Source: CAD feature listing. Evaluate the final solid. Frame: model axes, mm. A direction names the side the tool comes from. Round coordinates to 2 decimals unless told otherwise and drop trailing zeros. Order: outer loops, then holes, each group sorted by start corner. A loop starts at its lowest first (then second) coordinate and runs counter-clockwise, first axis right, second up. Notation, with made-up numbers: (52, -7) -> (108, -7) arc R19 cw to (108, 24) -> close; hole circle Ø8 at (-30, 86.5). An arc over 180 degrees is marked (long way). Write item = value, one per line. Start each with the question number.
(1) Cut plane B-B on x = 40. Return the cut outline in (y, z), then the cut area to 3 significant figures.
(2) Cut plane D-D on x = 12.5. Return the cut outline in (y, z).
(3) Cut plane C-C on z = -70. Return the cut outline in (x, y), then the cut area to 3 significant figures.
(4) Ray query, line 1 (Z direction, x = 40, y = 3); line 2 (Y direction, x = 5, z = -85); line 3 (Z direction, x = 17, y = 24). Return the intervals inside material, ascending.
(5) Contact query for flat-ended pins moving along their axis: pin 1 Ø6 at (x, z) = (40, -70) entering from +Y; pin 2 Ø8 at (x, z) = (24.5, -25.5) entering from -Y; pin 3 Ø1.5 at (x, z) = (39.5, -70) entering from -Y; pin 4 Ø10 at (y, z) = (35.5, -85.5) entering from +X. Output: stop coordinate, or through.
(6) Reachability of faces 1 (the face through (20, 5, -90)), 2 (the face through (25, 0, -49)) from +Z, -Z, +X, -X, +Y, -Y: full face, straight path, thin tool, end or side. Return the list, or none.
(7) Cut plane A-A on y = 4. Return the cut outline in (x, z).
(8) Draft query along X for faces 3 (the face through (42.31, 2.46, -70.96)), 4 (the face through (17.5, 2.5, -49.9)), 5 (the face through (50, 12, -49)), 6 (the face through (25, 12, -100)). Return one class per face: released by +X, released by -X, zero draft, split by the parting line, or undercut.
Autodesk Inventor part; units mm, degrees
ref_plane "Work Plane1" through (0, 55, 0) normal (0, 1, 0) x (1, 0, 0)
ref_plane "YZ Plane" through (0, 0, 0) normal (1, 0, 0) x (0, 1, 0)
ref_plane "XZ Plane" through (0, 0, 0) normal (0, 1, 0) x (-1, 0, 0)
sketch "Sketch1" plane through (0, 0, 0) normal (0, 1, 0) x (-1, 0, 0)
  line L0 (0, 0) -> (-50, 0)
  line L1 (-50, 0) -> (-50, -100)
  line L2 (-50, -100) -> (0, -100)
  line L3 (0, -100) -> (0, 0)
  dimension "d3" = 100
  dimension "d4" = 50
extrude "Extrusion1" add sketch "Sketch1" along normal blind 25
fillet "Fillet1" radius 2 1 edges at (25, 25, 0)
ref_plane "Work Plane1" through (0, 55, 0) normal (0, 1, 0) x (1, 0, 0)
sketch "Sketch2" plane through (0, 55, 0) normal (0, 1, 0) x (1, 0, 0)
  point P0 (0, 0)
sketch "Sketch3" plane through (0, 25, 0) normal (0, 1, 0) x (1, 0, 0)
  circle A0 centre (23.7799, 91.5707) radius 6.9252
  point P0 (0, 0)
sketch "Sketch4" plane through (0, 55, 0) normal (0, 1, 0) x (1, 0, 0)
  circle A0 centre (23.7424, 91.7378) radius 3.5123
  point P0 (0, 0)
loft "Loft1" add profiles "Sketch3", "Sketch4"
sketch "Sketch5" plane through (0, 0, 0) normal (0, -1, 0) x (1, 0, 0)
  line L0 (50, -100) -> (0, -100)
  line L1 (50, -100) -> (50, -90)
  line L2 (50, -2) -> (50, -100)
  line L3 (50, -90) -> (40, -90)
  circle A0 centre (40, -90) radius 2.5
  line L4 (40, -90) -> (40, -73.1599)
  line L5 (40, -90) -> (17.7006, -90)
  circle A1 centre (40, -70) radius 2.5
  circle A2 centre (40, -50) radius 2.5
  circle A3 centre (20, -90) radius 2.5
  circle A4 centre (20, -70) radius 2.5
  circle A5 centre (20, -50) radius 2.5
  point P0 (0, 0)
  dimension "d10" = 10
  dimension "d11" = 10
  dimension "d12" = 5
  dimension "d15" = 20
  dimension "d18" = 20
extrude "Extrusion2" cut sketch "Sketch5" against normal blind 5
properties part number "kappale"
Evaluation:
q1.outline = (0, -100) -> (25, -100) -> (25, -2) arc R2 ccw to (23, 0) -> (0, 0) -> (0, -47.5) -> (5, -47.5) -> (5, -52.5) -> (0, -52.5) -> (0, -67.5) -> (5, -67.5) -> (5, -72.5) -> (0, -72.5) -> (0, -87.5) -> (5, -87.5) -> (5, -92.5) -> (0, -92.5) -> close
q1.area = 2,420 mm^2
q2.outline = (0, -100) -> (25, -100) -> (25, -2) arc R2 ccw to (23, 0) -> (0, 0) -> close
q3.outline = (0, 0) -> (17.5, 0) -> (17.5, 5) -> (22.5, 5) -> (22.5, 0) -> (37.5, 0) -> (37.5, 5) -> (42.5, 5) -> (42.5, 0) -> (50, 0) -> (50, 25) -> (0, 25) -> close
q3.area = 1,200 mm^2
q4.line_1 = -100 to -92.5, -87.5 to -72.5, -67.5 to -52.5, -47.5 to 0
q4.line_2 = 0 to 25
q4.line_3 = -100 to -0.27
q5.pin_1 = 25
q5.pin_2 = 0
q5.pin_3 = 5
q5.pin_4 = 29.53
q6.face_1 = -Y
q6.face_2 = +Z, -Z, +X, -X, -Y
q7.outline = (0, -100) -> (50, -100) -> (50, 0) -> (0, 0) -> close; hole circle Ø5 at (20, -90); hole circle Ø5 at (20, -70); hole circle Ø5 at (20, -50); hole circle Ø5 at (40, -90); hole circle Ø5 at (40, -70); hole circle Ø5 at (40, -50)
q8.face_3 = undercut
q8.face_4 = undercut
q8.face_5 = released by +X
q8.face_6 = zero draft
